Design review of the part built by this model. Coordinates are the model's own, in mm. Face numbers are marked on the shaded views. A direction names the side the tool comes from. Give positions to 0.01 mm unless a question says otherwise; leave off trailing zeros. Loops run counter-clockwise (first coordinate to the right, second up) from the corner with the lowest first, then second, coordinate; pieces in that order, holes last. Notation, with made-up numbers: (21, 0) -> (75, 0) arc R18 ccw to (75, 17) -> close; hole circle Ø1 at (-4, 52). An arc over 180 degrees is marked (long way). Use a Markdown table: item, result. Add a question column.
1. Add section B-B (z = 4). Count the separate pieces of the cut face and the enclosed holes in it, and give its area (3 significant figures).
2. Draft analysis for pull direction Z (two halves, no side actions). For the marked faces 1, 2 and 3, state which applies: pulls with the +Z half, pulls with the -Z half, needs draft (parallel to the pull), parting line crosses it, or undercut.
3. Add section A-A (x = 5). State the section outline as (y, z) points.
4. For pin 1 Ø1.5 at (y, z) = (-7.5, 10) entering from +X; pin 2 Ø12 at (x, z) = (14.5, -21.5) entering from -Y; pin 3 Ø3 at (x, y) = (12.5, 8.5) entering from +Z, all flat-tipped, find the tip position at first contact; note any pin that passes through.
5. For the marked faces 4 and 5, list the 3-axis set-ups (+Z, -Z, +X, -X, +Y, -Y) from which the entire face can be reached by the end or side of a thin tool; tool diameter is ignored.
6. To check wall thickness, follow line 1 (Z direction, x = 0.2, y = 0); line 2 (X direction, y = -5.5, z = 1); line 3 (Z direction, x = 2, y = 0). State the ranges of each line that lie inside material, in increasing order.
7. Add section C-C (x = 17.5). State the section outline as (y, z) points, and give its area (3 significant figures).
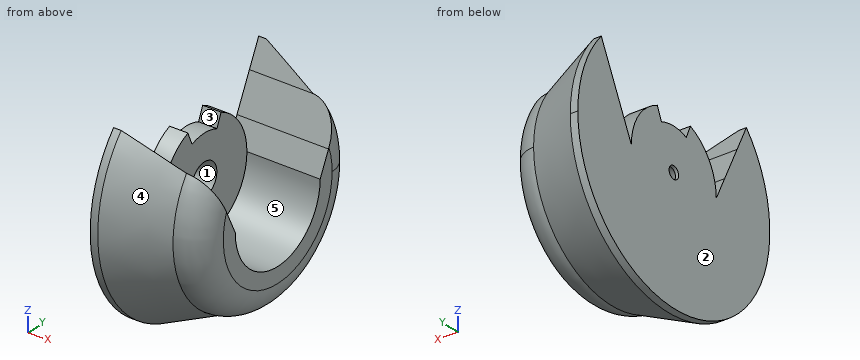
```python
from build123d import *

# Parameters (mm, degrees)
F1_DEPTH       = 20
F2_DEPTH       = 20
F3_R           = 6.3
F4_DEPTH       = 14
F5_S5_R        = 21.6830909865
F5_T6_DEPTH    = 40
F6_DEPTH       = 4
F7_DEPTH       = 25
F9_D           = 2.7
F9_DEPTH       = 12
F9_CSINK_D     = 7
F9_CSINK_ANGLE = 66
F9_TIP         = 0.8111618357


# Not quite as in the source:
# - a fillet or chamfer that OpenCascade refuses, or shapes differently, is made with other operations: its cross-section is extruded or revolved along the edge and cut away or added


with BuildPart() as f1:
    # F0 (on Right) → F1 (new body)
    with BuildSketch(Plane.YZ):
        with BuildLine():
            ThreePointArc((4.6887735419, 11.0460582414), (10.0066298648, 6.6232438237), (12, 0))
            Line((12, 0), (14.3613430429, 4.925409334))
            ThreePointArc((14.3613430429, 4.925409334), (0, 15.1824843522), (-14.3613430429, 4.925409334))
            Line((-14.3613430429, 4.925409334), (-12, 0))
            ThreePointArc((-12, 0), (-10.0066298648, 6.6232438237), (-4.6887735419, 11.0460582414))
            ThreePointArc((-4.6887735419, 11.0460582414), (0, 12), (4.6887735419, 11.0460582414))
        make_face()
        with BuildLine():
            Line((14.3613430429, 4.925409334), (12, 0))
            ThreePointArc((12, 0), (0, -12), (-12, 0))
            Line((-12, 0), (-14.3613430429, 4.925409334))
            ThreePointArc((-14.3613430429, 4.925409334), (-2.4966943224, -14.9757920847), (15.1824843522, 0))
            ThreePointArc((15.1824843522, 0), (14.9757920847, 2.4966943224), (14.3613430429, 4.925409334))
        make_face()
    extrude(amount=F1_DEPTH)

    # F0 (on Right) → F2 (join)
    with BuildSketch(Plane.YZ):
        with BuildLine():
            ThreePointArc((-14.3613430429, 4.925409334), (0, 15.1824843522), (14.3613430429, 4.925409334))
            Line((14.3613430429, 4.925409334), (17.8804215677, 12.2656821778))
            ThreePointArc((17.8804215677, 12.2656821778), (13.0689294726, 17.30200905), (6.9088656071, 20.5529562533))
            Line((6.9088656071, 20.5529562533), (-6.9088656071, 20.5529562533))
            ThreePointArc((-6.9088656071, 20.5529562533), (-13.0689294726, 17.30200905), (-17.8804215677, 12.2656821778))
            Line((-17.8804215677, 12.2656821778), (-14.3613430429, 4.925409334))
        make_face()
        with BuildLine():
            Line((17.8804215677, 12.2656821778), (14.3613430429, 4.925409334))
            ThreePointArc((14.3613430429, 4.925409334), (14.9757920847, 2.4966943224), (15.1824843522, 0))
            ThreePointArc((15.1824843522, 0), (-2.4966943224, -14.9757920847), (-14.3613430429, 4.925409334))
            Line((-14.3613430429, 4.925409334), (-17.8804215677, 12.2656821778))
            ThreePointArc((-17.8804215677, 12.2656821778), (-6.4208109689, -20.710616148), (21.6830909865, 0))
            ThreePointArc((21.6830909865, 0), (20.710616148, 6.4208109689), (17.8804215677, 12.2656821778))
        make_face()
        with BuildLine():
            Line((-6.9088656071, 20.5529562533), (6.9088656071, 20.5529562533))
            ThreePointArc((6.9088656071, 20.5529562533), (0, 21.6830909865), (-6.9088656071, 20.5529562533))
        make_face()
    extrude(amount=F2_DEPTH)

    # F3
    f3_edges = [f1.edges().sort_by_distance(p)[0] for p in [
        (20, -6.908866, -20.552956),
    ]]
    fillet(f3_edges, radius=F3_R)

    # F0 (on Right) → F4 (join)
    with BuildSketch(Plane.YZ):
        with BuildLine():
            ThreePointArc((6.9088656071, 20.5529562533), (13.0689294726, 17.30200905), (17.8804215677, 12.2656821778))
            Line((17.8804215677, 12.2656821778), (20.5131543573, 17.7571700385))
            ThreePointArc((20.5131543573, 17.7571700385), (19.1631742939, 19.2062318127), (17.7110863222, 20.5529562533))
            Line((17.7110863222, 20.5529562533), (6.9088656071, 20.5529562533))
        make_face()
        with BuildLine():
            ThreePointArc((-6.9088656071, 20.5529562533), (0, 21.6830909865), (6.9088656071, 20.5529562533))
            Line((6.9088656071, 20.5529562533), (17.7110863222, 20.5529562533))
            ThreePointArc((17.7110863222, 20.5529562533), (0, 27.1312843312), (-17.7110863222, 20.5529562533))
            Line((-17.7110863222, 20.5529562533), (-6.9088656071, 20.5529562533))
        make_face()
        with BuildLine():
            Line((-20.5131543573, 17.7571700385), (-17.8804215677, 12.2656821778))
            ThreePointArc((-17.8804215677, 12.2656821778), (-13.0689294726, 17.30200905), (-6.9088656071, 20.5529562533))
            Line((-6.9088656071, 20.5529562533), (-17.7110863222, 20.5529562533))
            ThreePointArc((-17.7110863222, 20.5529562533), (-19.1631742939, 19.2062318127), (-20.5131543573, 17.7571700385))
        make_face()
        with BuildLine():
            Line((20.5131543573, 17.7571700385), (17.8804215677, 12.2656821778))
            ThreePointArc((17.8804215677, 12.2656821778), (20.710616148, 6.4208109689), (21.6830909865, 0))
            ThreePointArc((21.6830909865, 0), (-6.4208109689, -20.710616148), (-17.8804215677, 12.2656821778))
            Line((-17.8804215677, 12.2656821778), (-20.5131543573, 17.7571700385))
            ThreePointArc((-20.5131543573, 17.7571700385), (-9.4751877571, -25.4229700552), (27.1312843312, 0))
            ThreePointArc((27.1312843312, 0), (25.4229700552, 9.4751877571), (20.5131543573, 17.7571700385))
        make_face()
    extrude(amount=F4_DEPTH)

    # F5: chamfer of 5.5 x 12.3532022565 on 1 edges, made by hand


with BuildPart() as f5_tool2:
    # F5_s3 → F5_t4 (revolve)
    with BuildSketch(Plane(origin=(0, 0, 0), x_dir=(1, 0, 0), z_dir=(0, 0.6544905808, 0.7560701553))):
        Polygon((14, -21.6312843312), (1.6467977435, -27.1312843312), (14, -27.1312843312), align=None)
    revolve(axis=Axis((14, 0, 0), (1, 0, 0)))

    # F5_s5 → F5_t6 (cut, symmetric)
    with BuildSketch(Plane.YZ.offset(7.8)):
        Circle(F5_S5_R)
    extrude(amount=F5_T6_DEPTH, both=True, mode=Mode.SUBTRACT)


with BuildPart() as f1_1:
    add(f1.part)

    # F5_t1: cut F5_tool2
    add(f5_tool2.part, mode=Mode.SUBTRACT)

    # F0 (on Right) → F6 (join)
    with BuildSketch(Plane.YZ):
        with BuildLine():
            ThreePointArc((-12, 0), (0, -12), (12, 0))
            ThreePointArc((12, 0), (10.0066298648, 6.6232438237), (4.6887735419, 11.0460582414))
            Line((4.6887735419, 11.0460582414), (3.5165801564, 8.2845436811))
            ThreePointArc((3.5165801564, 8.2845436811), (7.5049723986, 4.9674328678), (9, 0))
            ThreePointArc((9, 0), (-4.9674328678, -7.5049723986), (-3.5165801564, 8.2845436811))
            Line((-3.5165801564, 8.2845436811), (-4.6887735419, 11.0460582414))
            ThreePointArc((-4.6887735419, 11.0460582414), (-10.0066298648, 6.6232438237), (-12, 0))
        make_face()
        with BuildLine():
            ThreePointArc((9, 0), (7.5049723986, 4.9674328678), (3.5165801564, 8.2845436811))
            Line((3.5165801564, 8.2845436811), (0, 0))
            Line((0, 0), (-3.5165801564, 8.2845436811))
            ThreePointArc((-3.5165801564, 8.2845436811), (-4.9674328678, -7.5049723986), (9, 0))
        make_face()
        with BuildLine():
            Line((0, 0), (3.5165801564, 8.2845436811))
            ThreePointArc((3.5165801564, 8.2845436811), (0, 9), (-3.5165801564, 8.2845436811))
            Line((-3.5165801564, 8.2845436811), (0, 0))
        make_face()
    extrude(amount=F6_DEPTH)

    # F0 (on Right) → F7 (cut)
    with BuildSketch(Plane.YZ):
        with BuildLine():
            ThreePointArc((4.6887735419, 11.0460582414), (10.0066298648, 6.6232438237), (12, 0))
            Line((12, 0), (14.3613430429, 4.925409334))
            ThreePointArc((14.3613430429, 4.925409334), (0, 15.1824843522), (-14.3613430429, 4.925409334))
            Line((-14.3613430429, 4.925409334), (-12, 0))
            ThreePointArc((-12, 0), (-10.0066298648, 6.6232438237), (-4.6887735419, 11.0460582414))
            ThreePointArc((-4.6887735419, 11.0460582414), (0, 12), (4.6887735419, 11.0460582414))
        make_face()
        with BuildLine():
            ThreePointArc((-14.3613430429, 4.925409334), (0, 15.1824843522), (14.3613430429, 4.925409334))
            Line((14.3613430429, 4.925409334), (17.8804215677, 12.2656821778))
            ThreePointArc((17.8804215677, 12.2656821778), (13.0689294726, 17.30200905), (6.9088656071, 20.5529562533))
            Line((6.9088656071, 20.5529562533), (-6.9088656071, 20.5529562533))
            ThreePointArc((-6.9088656071, 20.5529562533), (-13.0689294726, 17.30200905), (-17.8804215677, 12.2656821778))
            Line((-17.8804215677, 12.2656821778), (-14.3613430429, 4.925409334))
        make_face()
        with BuildLine():
            Line((-6.9088656071, 20.5529562533), (6.9088656071, 20.5529562533))
            ThreePointArc((6.9088656071, 20.5529562533), (0, 21.6830909865), (-6.9088656071, 20.5529562533))
        make_face()
        with BuildLine():
            ThreePointArc((-6.9088656071, 20.5529562533), (0, 21.6830909865), (6.9088656071, 20.5529562533))
            Line((6.9088656071, 20.5529562533), (17.7110863222, 20.5529562533))
            ThreePointArc((17.7110863222, 20.5529562533), (0, 27.1312843312), (-17.7110863222, 20.5529562533))
            Line((-17.7110863222, 20.5529562533), (-6.9088656071, 20.5529562533))
        make_face()
        with BuildLine():
            Line((-20.5131543573, 17.7571700385), (-17.8804215677, 12.2656821778))
            ThreePointArc((-17.8804215677, 12.2656821778), (-13.0689294726, 17.30200905), (-6.9088656071, 20.5529562533))
            Line((-6.9088656071, 20.5529562533), (-17.7110863222, 20.5529562533))
            ThreePointArc((-17.7110863222, 20.5529562533), (-19.1631742939, 19.2062318127), (-20.5131543573, 17.7571700385))
        make_face()
        with BuildLine():
            ThreePointArc((6.9088656071, 20.5529562533), (13.0689294726, 17.30200905), (17.8804215677, 12.2656821778))
            Line((17.8804215677, 12.2656821778), (20.5131543573, 17.7571700385))
            ThreePointArc((20.5131543573, 17.7571700385), (19.1631742939, 19.2062318127), (17.7110863222, 20.5529562533))
            Line((17.7110863222, 20.5529562533), (6.9088656071, 20.5529562533))
        make_face()
    extrude(amount=F7_DEPTH, mode=Mode.SUBTRACT)

    # F9
    with Locations(Plane.YZ.offset(4)):
        with Locations((0, -0.2123973536)):
            CounterSinkHole(F9_D / 2, F9_CSINK_D / 2, depth=F9_DEPTH, counter_sink_angle=F9_CSINK_ANGLE)
            with Locations((0, 0, -(F9_DEPTH + F9_TIP / 2))):  # 118° drill point
                Cone(0, F9_D / 2, F9_TIP, mode=Mode.SUBTRACT)


solid = f1_1.part
```
Taken from the geometry:
| question | item | result |
|---|---|---|
| 1 | separate pieces | 3 |
| 1 | enclosed holes | 0 |
| 1 | area | 455 mm^2 |
| 2 | face 1 | undercut |
| 2 | face 2 | needs draft |
| 2 | face 3 | pulls with the +Z half |
| 3 | outline | (-19.81, 16.28) arc R25.64 ccw (long way) to (19.81, 16.28) -> (12, 0) arc R12 cw to (-12, 0) -> close |
| 4 | pin 1 | stops at x = 4 |
| 4 | pin 2 | stops at y = -15.86 |
| 4 | pin 3 | stops at z = -6.63 |
| 5 | face 4 | +X |
| 5 | face 5 | +Z, +X |
| 6 | line 1 | z = -27.13 to -1.56, 1.14 to 9 |
| 6 | line 2 | x = 0 to 4 |
| 6 | line 3 | z = -26.97 to -2.41, 1.99 to 9 |
| 7 | outline | (-17.24, 10.92) arc R20.41 ccw (long way) to (17.24, 10.92) -> (12, 0) arc R12 cw to (-12, 0) -> close |
| 7 | area | 532 mm^2 |
